Geometry check sheet. Reference: the model listing, model coordinates, mm. A direction names the side the tool comes from. Give positions to 0.01 mm unless a question says otherwise; leave off trailing zeros. Loops run counter-clockwise (first coordinate to the right, second up) from the corner with the lowest first, then second, coordinate; pieces in that order, holes last. Notation, with made-up numbers: (-16, 36.25) - (11, 36.25) arc R21 ccw to (11, 59.25) - close; hole circle Ø10 at (28, 72). An arc over 180 degrees is marked (long way). One line per question, with ' | ' between items. Start each with the question number.
Autodesk Inventor part; units mm, degrees
ref_plane "YZ Plane" through (0, 0, 0) normal (1, 0, 0) x (0, 1, 0)
ref_plane "XZ Plane" through (0, 0, 0) normal (0, 1, 0) x (-1, 0, 0)
ref_plane "XY Plane" through (0, 0, 0) normal (0, 0, 1) x (1, 0, 0)
sketch "Sketch1" plane through (0, 0, 0) normal (0, 0, 1) x (1, 0, 0)
  line L0 (0, 0) -> (0, 16.5)
  line L1 (0, 16.5) -> (-10, 16.5)
  line L2 (-10, 16.5) -> (-26.5, 20.348)
  line L3 (-26.5, 20.348) -> (-36.5, 20.348)
  line L4 (-36.5, 20.348) -> (-36.5, 3.848)
  line L5 (-36.5, 3.848) -> (-26.5, 3.848)
  line L6 (-26.5, 3.848) -> (-10, 0)
  line L7 (-10, 0) -> (0, 0)
  dimension "d0" = 10
  dimension "d1" = 10
  dimension "d2" = 10
  dimension "d3" = 10
  dimension "d4" = 3.848
  dimension "d5" = 36.5
  dimension "d6" = 16.5
extrude "Extrusion1" add sketch "Sketch1" along normal blind 1.6
sketch "Sketch2" plane through (0, 0, 1.6) normal (0, 0, 1) x (1, 0, 0)
  line L0 (-7.4638, 8.25) -> (0, 8.25)
  line L1 (0, 0) -> (0, 16.5)
  line L2 (-36.5, 20.348) -> (-36.5, 3.848)
  line L3 (-36.5, 12.098) -> (-30.2249, 12.098)
  line L4 (-26.5, 20.348) -> (-36.5, 20.348)
  line L5 (-31.9735, 20.348) -> (-31.9735, 3.848)
  line L6 (-4.5265, 16.5) -> (-4.5265, 0)
  line L7 (-10, 0) -> (0, 0)
  line L8 (0, 16.5) -> (-10, 16.5)
  dimension "d9" = 16.5
  dimension "d12" = 27.447
  dimension "d13" = 36.5
  dimension "d14" = 4.5265
fillet "Fillet1" radius 1 4 edges at (-36.5, 20.348, 0.8) (-36.5, 3.848, 0.8) (0, 0, 0.8) (0, 16.5, 0.8)
sketch "OUTLINE" plane through (0, 0, 1.6) normal (0, 0, 1) x (1, 0, 0)
  arc A0 (0, 15.5) -> (-1, 16.5) centre (-1, 15.5) ccw
  line L0 (-1, 16.5) -> (-10, 16.5)
  line L1 (-10, 16.5) -> (-26.5, 20.348)
  line L2 (-26.5, 20.348) -> (-35.5, 20.348)
  arc A1 (-35.5, 20.348) -> (-36.5, 19.348) centre (-35.5, 19.348) ccw
  line L3 (-36.5, 19.348) -> (-36.5, 4.848)
  arc A2 (-36.5, 4.848) -> (-35.5, 3.848) centre (-35.5, 4.848) ccw
  line L4 (-35.5, 3.848) -> (-26.5, 3.848)
  line L5 (-26.5, 3.848) -> (-10, 0)
  line L6 (-10, 0) -> (-1, 0)
  arc A3 (-1, 0) -> (0, 1) centre (-1, 1) ccw
  line L7 (0, 1) -> (0, 15.5)
  point P0 (0, 0)
sketch "EXTRA" plane through (0, 0, 1.6) normal (0, 0, 1) x (1, 0, 0)
  circle A0 centre (-3.0265, 2.25) radius 0.49
  circle A1 centre (-6.0265, 14.25) radius 0.49
  circle A2 centre (-30.4735, 6.098) radius 0.5193
  circle A3 centre (-33.4735, 18.098) radius 0.5193
  circle A4 centre (-6.0265, 2.25) radius 0.49
  circle A5 centre (-3.0265, 14.25) radius 0.49
  circle A6 centre (-30.4735, 18.098) radius 0.49
  circle A7 centre (-33.4735, 6.098) radius 0.49
  point P0 (0, 0)
equation "\"d1\" = d0"
equation "\"d2\" = d1"
equation "\"d3\" = d0"
equation "\"d14\" = -0.5 * d12 + 0.5 * d13"
properties part number "DB2_Bridge"
(1) Section check C-C, the plane y = 1.5. Record the boundary of the cut face in (x, z), and give its area (3 significant figures).
(2) Tool access check on faces 1 (the face through (-31, 3.848, 1)), 2 (the face through (-5, 16.5, 1)), 3 (the face through (-0.301, 0.285, 0.811)). Record the directions out of +Z, -Z, +X, -X, +Y, -Y that give a thin tool (end or side, any length) a straight path to the whole face; none if there is none.
(3) Section check B-B, the plane x = -3. Record the boundary of the cut face in (y, z).
(4) Material ranges on line 1 (Y direction, x = -6.5, z = 0.3); line 2 (Y direction, x = -29.5, z = 0.55); line 3 (X direction, y = 16, z = 0.3), recorded low to high.
(5) Section check A-A, the plane z = 1.15. Record the boundary of the cut face in (x, y).
(6) Depth check by flat-ended pin: pin 1 Ø0.8 at (x, z) = (-7, 0.5) entering from +Y; pin 2 Ø0.8 at (x, z) = (-30, 1) entering from -Y. Enter the tip coordinate at first touch or a pass-through.
Numbers:
1) outline: (-16.43, 0) - (0, 0) - (0, 1.6) - (-16.43, 1.6) - close | area: 26.3 mm^2
2) face 1: +Z, -Z, -X, -Y | face 2: +Z, -Z, +X, +Y | face 3: +Z, -Z, +X, -Y
3) outline: (0, 0) - (16.5, 0) - (16.5, 1.6) - (0, 1.6) - close
4) line 1: 0 to 16.5 | line 2: 3.85 to 20.35 | line 3: -36.5 to -0.13
5) outline: (-36.5, 4.85) arc R1 ccw to (-35.5, 3.85) - (-26.5, 3.85) - (-10, 0) - (-1, 0) arc R1 ccw to (0, 1) - (0, 15.5) arc R1 ccw to (-1, 16.5) - (-10, 16.5) - (-26.5, 20.35) - (-35.5, 20.35) arc R1 ccw to (-36.5, 19.35) - close
6) pin 1: y = 16.5 | pin 2: y = 3.85
